Could you check a few things on this model? Use its own coordinates, in mm. A direction names the side the tool comes from. Coordinates: 2 decimals unless noted, no trailing zeros. Loops run counter-clockwise (first coordinate to the right, second up) from the corner with the lowest first, then second, coordinate; pieces in that order, holes last. Notation, with made-up numbers: M -13.5,63 L 2.5,63 A18 cw 2.5,80 Z; hole C 12.25,77 d5. An arc over 180 degrees is marked long. Use one line per item in the form item = value. Start each with the question number.
```python
from build123d import *


with BuildPart() as part:
    # BodySke → BaseBody (revolve)
    with BuildSketch(Plane.XY, mode=Mode.PRIVATE) as basebody_sk:
        with BuildLine():
            Line((0, 0), (0, 4.02336))
            Line((0, 4.02336), (0.00508, 4.02336))
            Line((0.00508, 4.02336), (0.00508, 4.02844))
            ThreePointArc((0.00508, 4.02844), (0.23114, 4.2545), (0.4572, 4.02844))
            Line((0.4572, 4.02844), (0.4572, 3.71475))
            Line((0.4572, 3.71475), (0.6858, 3.71475))
            Line((0.6858, 3.71475), (0.6858, 3.4544))
            Line((0.6858, 3.4544), (1.518354809, 3.4544))
            Line((1.518354809, 3.4544), (2.286, 3.175))
            Line((2.286, 3.175), (17.149163308, 3.175))
            Line((17.149163308, 3.175), (19.05, 2.2479))
            Line((19.05, 2.2479), (19.05, 0))
            Line((19.05, 0), (0, 0))
        make_face()
    revolve(basebody_sk.sketch.rotate(Axis((0, 0, 0), (1, 0, 0)), 90), axis=Axis((0, 0, 0), (1, 0, 0)))


solid = part.part
```
Item 1: I want a section at A-A (z = 0). Write out the boundary of the cut face in (x, y) (3 decimals).
Item 2: Please list where these lines run through material, in increasing order: line 1 along X through (y, z) = (1.75, 3.5); line 2 along Z through (x, y) = (2, 0.75); line 3 along Y through (x, z) = (14.25, -1).
Item 3: I'm going to push flat-ended pins straight in: P1, Ø1.5, axis at y = 0.5, z = 3, coming from the +X side; P2, Ø4, axis at x = 7.5, y = 3, coming from the +Z side; P3, Ø1, axis at x = 12, y = 3, coming from the +Z side. Where does each tip first touch, or does it pass through?
Item 4: I want a section at C-C (x = 5.75). Write out the boundary of the cut face in (y, z) (3 decimals).
Item 5: For faces 1 (the flat face through (19.05, 0, 0)), 2 (the cylindrical face through (9.82, 1.93, -2.52)), which set-ups out of +Z, -Z, +X, -X, +Y, -Y let a thin tool reach every point of the face, with its end or its side?
Item 6: I want a section at D-D (x = 17.75). Write out the boundary of the cut face in (y, z).
Worked answers:
q1.outline = M 0,-4.023 L 0.005,-4.023 L 0.005,-4.028 A0.226 ccw 0.457,-4.028 L 0.457,-3.715 L 0.686,-3.715 L 0.686,-3.454 L 1.518,-3.454 L 2.286,-3.175 L 17.149,-3.175 L 19.05,-2.248 L 19.05,2.248 L 17.149,3.175 L 2.286,3.175 L 1.518,3.454 L 0.686,3.454 L 0.686,3.715 L 0.457,3.715 L 0.457,4.028 A0.226 ccw 0.005,4.028 L 0.005,4.023 L 0,4.023 Z
q2.line_1 = 0 to 0.46
q2.line_2 = -3.19 to 3.19
q2.line_3 = -3.01 to 3.01
q3.P1 = 18.96
q3.P2 = 3.01
q3.P3 = 1.96
q4.outline = C 0,0 d6.35
q5.face_1 = +Z, -Z, +X, +Y, -Y
q5.face_2 = +X
q6.outline = C 0,0 d5.76
